Could you check a few things on this model? Use its own coordinates, in mm. A direction names the side the tool comes from. Give positions to 0.01 mm unless a question says otherwise; leave off trailing zeros. Loops run counter-clockwise (first coordinate to the right, second up) from the corner with the lowest first, then second, coordinate; pieces in that order, holes last. Notation, with made-up numbers: M 52,-16.5 L 73,-16.5 A10 cw 73,-2.5 Z; hole C 54,58 d8. An arc over 180 degrees is marked long. Use CSV: the item, a comma, the result in double quotes.
```python
from build123d import *

# Parameters (mm, degrees)
F0_R     = 6.4
F1_DEPTH = 50
F4_R     = 4.4
F5_DEPTH = 50.001
F6_SIZE  = 1.99999


# Not quite as in the source:
# - a fillet or chamfer is up to 0.001 mm smaller than in the source, because OpenCascade refuses the exact size


with BuildPart() as f1:
    # F0 (on Right) → F1 (new body)
    with BuildSketch(Plane.YZ):
        Circle(F0_R)
    extrude(amount=F1_DEPTH)

    # F2 (on Front) → F3 (revolve)
    with BuildSketch(Plane.XZ):
        Polygon((10, 0), (10, 7.5), (0, 0), align=None)
        Polygon((20, 0), (20, 7.5), (10, 0), align=None)
        Polygon((40, 0), (30, 7.5), (30, 0), align=None)
        Polygon((50, 0), (40, 7.5), (40, 0), align=None)
    revolve(axis=Axis((25, 0, 0), (1, 0, 0)))

    # F4 (on face) → F5 (cut, through all)
    with BuildSketch(Plane(origin=(0, 0, 0), x_dir=(0, -1, 0), z_dir=(-1, 0, 0))):
        Circle(F4_R)
    extrude(amount=-F5_DEPTH, mode=Mode.SUBTRACT)

    # F6 (size 2 in the source; OpenCascade refuses exactly that, so slightly less here)
    f6_edges = [f1.edges().sort_by_distance(p)[0] for p in [
        (50, -6.4, 0),
        (0, -6.4, 0),
    ]]
    chamfer(f6_edges, length=F6_SIZE)


solid = f1.part
```
1. Please list where these lines run through material, in increasing order: line 1 (X direction, y = 5, z = 4.75); line 2 (X direction, y = -5.5, z = -3.5); line 3 (Z direction, x = 32, y = 0).
Outcome:
line 1,"9.2 to 10, 19.2 to 20, 30 to 30.8, 40 to 40.8"
line 2,"8.69 to 10, 18.69 to 20, 30 to 31.31, 40 to 41.31"
line 3,"-6.4 to -4.4, 4.4 to 6.4"
2. I want a section at B-B, the plane x = 40.5. List the corners of the cut face in (y, z) for me (3 decimals), then the cut area to 3 significant figures.
Outcome:
outline,"C 0,0 d14.25; hole C 0,0 d8.8"
area,"98.7 mm2"
3. If we mould it in two halves opening along Z, with no side actions, what happens to faces 1 (the face through (5.22, -5.08, -3.89)), 2 (the face through (10, -3, -6)), 3 (the face through (24.65, -4.197, 1.322))? For each: +Z half, -Z half, draft (parallel to the pull), parting line (faces both ways), or undercut.
Outcome:
face 1,"parting line"
face 2,"draft"
face 3,"undercut"
4. I'm going to push flat-ended pins straight in: pin 1 Ø6 at (y, z) = (5, -4.5) entering from +X; pin 2 Ø5 at (x, z) = (14, -1.5) entering from -Y; pin 3 Ø6 at (x, y) = (15, -5) entering from -Z; pin 4 Ø1 at (y, z) = (-2, 4.5) entering from -X. Where does each tip first touch, or does it pass through?
Outcome:
pin 1,"x = 50"
pin 2,"y = -6.4"
pin 3,"z = -6.08"
pin 4,"x = 0.02"
5. I want a section at A-A, the plane x = 21.5. List the corners of the cut face in (y, z) for me.
Outcome:
outline,"C 0,0 d12.8; hole C 0,0 d8.8"
6. Which directions (+Z, -Z, +X, -X, +Y, -Y) give clear straight access to the entire face, cutting with the end or side of a thin tool? Please do faces 4 (the face through (24.93, -5.08, -3.89)), 5 (the face through (44.69, -5.08, -3.89)).
Outcome:
face 4,"none"
face 5,"+X"
